Model file for the job. Use its own axes, mm. Face numbers are marked on the shaded views. A direction names the side the tool comes from. Round coordinates to 2 decimals unless told otherwise and drop trailing zeros. Loops run counter-clockwise (first coordinate to the right, second up) from the corner with the lowest first, then second, coordinate; pieces in that order, holes last. Notation, with made-up numbers: M 58,85.25 L 85,85.25 A21 ccw 85,123.25 Z; hole C 11,-3.75 d9. An arc over 180 degrees is marked long. Answer in a Markdown table with one row per item.
from build123d import *

# Parameters (mm, degrees)
BOSS_EXTRUDE1_DEPTH      = 25
BOSS_EXTRUDE1_DEPTH_BACK = 25
SKETCH1_W                = 175
SKETCH1_H                = 50
SKETCH2_W                = 20
SKETCH2_H                = 50
CUT_EXTRUDE1_DEPTH       = 104.832798286
FILLET2_R                = 25
SKETCH3_W                = 56.175036023
SKETCH3_H                = 20
CUT_EXTRUDE2_DEPTH       = 104.832798286
FILLET6_R                = 25
HOLE1_D                  = 20
HOLE2_D                  = 20


with BuildPart() as part:
    # Sketch1 → Boss-Extrude1 (new, two sides: drawn at the far end of the back side and taken through both)
    with BuildSketch(Plane(origin=(0, 0, 0), x_dir=(0, 0, -1), z_dir=(1, 0, 0)).offset(-BOSS_EXTRUDE1_DEPTH_BACK)):
        Rectangle(SKETCH1_W, SKETCH1_H)
    extrude(amount=BOSS_EXTRUDE1_DEPTH + BOSS_EXTRUDE1_DEPTH_BACK)

    # Sketch2 → Cut-Extrude1 (cut, through all)
    with BuildSketch(Plane(origin=(0, 25, 0), x_dir=(1, 0, 0), z_dir=(0, 1, 0))):
        with Locations((0, -62.5)):
            Rectangle(SKETCH2_W, SKETCH2_H)
    extrude(amount=-CUT_EXTRUDE1_DEPTH, mode=Mode.SUBTRACT)

    # Fillet2
    fillet2_edges = [part.edges().sort_by_distance(p)[0] for p in [
        (-17.5, 25, 87.5),
        (17.5, 25, 87.5),
        (-17.5, -25, 87.5),
        (17.5, -25, 87.5),
    ]]
    fillet(fillet2_edges, radius=FILLET2_R - 0.0001)  # a hair under: the kernel refuses the full size

    # Sketch3 → Cut-Extrude2 (cut, through all)
    with BuildSketch(Plane(origin=(25, 0, 0), x_dir=(0, 0, -1), z_dir=(1, 0, 0))):
        with Locations((78.087518012, 0)):
            Rectangle(SKETCH3_W, SKETCH3_H)
    extrude(amount=-CUT_EXTRUDE2_DEPTH, mode=Mode.SUBTRACT)

    # Fillet6
    fillet6_edges = [part.edges().sort_by_distance(p)[0] for p in [
        (25, 17.5, -87.5),
        (25, -17.5, -87.5),
        (-25, -17.5, -87.5),
        (-25, 17.5, -87.5),
    ]]
    fillet(fillet6_edges, radius=FILLET6_R - 0.0001)  # a hair under: the kernel refuses the full size

    # Hole1 (through all)
    with Locations(Plane(origin=(0, 25, 0), x_dir=(1, 0, 0), z_dir=(0, 1, 0))):
        with Locations((0, 62.5)):
            Hole(HOLE1_D / 2)

    # Hole2 (through all)
    with Locations(Plane.ZY.offset(25)):
        with Locations((62.5, 0)):
            Hole(HOLE2_D / 2)


solid = part.part
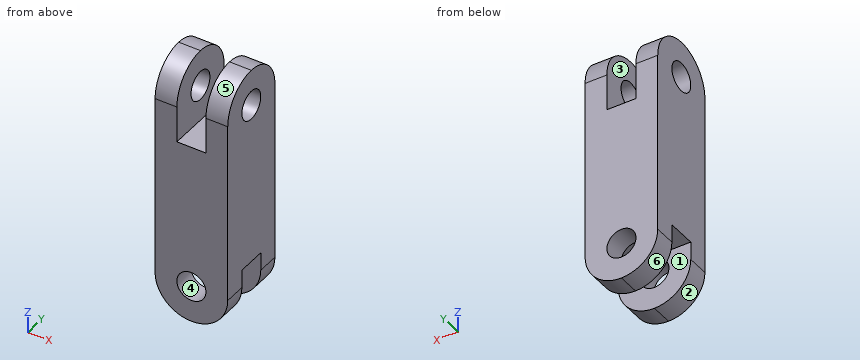
1. Pin check, flat tips, straight feed: pin 1 (6 mm diameter, centred on x = 6.5, y = -2, fed in from -Z); pin 2 (5 mm diameter, centred on x = 19, y = -15, fed in from -Z); pin 3 (12 mm diameter, centred on x = 0, z = -62.5, fed in from -Y); pin 4 (1.5 mm diameter, centred on x = -15, y = 12.5, fed in from -Z). Stop position of each tip, or through.
Verdict:
| item | result |
|---|---|
| pin 1 | stops at z = -50 |
| pin 2 | stops at z = -81.28 |
| pin 3 | passes through |
| pin 4 | stops at z = -83.04 |
2. Wall check: probe 1 along Z at (x, y) = (0, -16.5); probe 2 along X at (y, z) = (-20, 47.5). Give the ranges that are in metal, low to high.
Verdict:
| item | result |
|---|---|
| probe 1 | z = -87.5 to -72.5, -52.5 to 37.5 |
| probe 2 | x = -25 to -10, 10 to 25 |
3. Tool access for the marked faces 1, 2 and 3: list every direction of +Z, -Z, +X, -X, +Y, -Y with a clear straight run to the whole face (end or side of a thin tool).
Verdict:
| item | result |
|---|---|
| face 1 | -Z, +X, -X |
| face 2 | -Z, -X, +Y, -Y |
| face 3 | +Z, +Y, -Y |
4. Saw through at D-D (z = -57). Write the cut outline in (x, y).
Verdict:
| item | result |
|---|---|
| outline | M -25,-25 L -8.35,-25 L -8.35,-10 L -25,-10 Z; M -25,10 L -8.35,10 L -8.35,25 L -25,25 Z; M 8.35,-25 L 25,-25 L 25,-10 L 8.35,-10 Z; M 8.35,10 L 25,10 L 25,25 L 8.35,25 Z |
5. Mould opens along X. For the marked faces 4, 5 and 6 say: +X half, -X half, draft (parallel to the pull), parting line (faces both ways), or undercut.
Verdict:
| item | result |
|---|---|
| face 4 | undercut |
| face 5 | draft |
| face 6 | -X half |
6. Saw through at A-A (x = -6). Write the cut outline in (y, z), and give its area (3 significant figures).
Verdict:
| item | result |
|---|---|
| outline | M -25,-86.77 L -10,-86.77 L -10,-70.5 L -25,-70.5 Z; M -25,-54.5 L -10,-54.5 L -10,-50 L 10,-50 L 10,-54.5 L 25,-54.5 L 25,37.5 L -25,37.5 Z; M 10,-86.77 L 25,-86.77 L 25,-70.5 L 10,-70.5 Z |
| area | 5,000 mm² |
